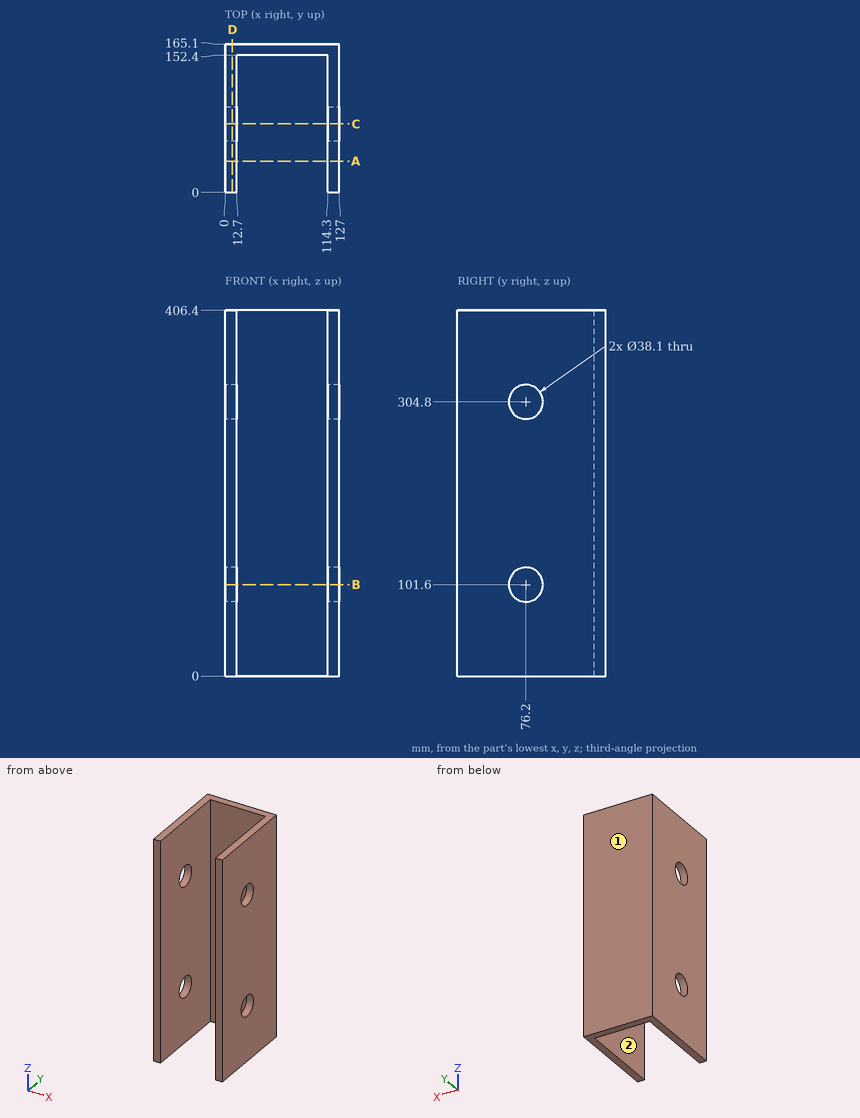
Study the drawing (mm; zero at the part's minimum x, y, z) and answer. A direction names the side the tool comes from. Give positions to 0.01 mm unless a question says otherwise; leave off trailing zeros. Loops run counter-clockwise (first coordinate to the right, second up) from the corner with the lowest first, then second, coordinate; pieces in that order, holes last. Notation, with made-up numbers: M 81.25,83 L 106.25,83 A9 cw 106.25,93 Z; hole C 73,66 d6. An arc over 180 degrees is marked long. Use CSV: the item, a comma, the result in double quotes.
1) Find section C-C on y = 76.2. Write down the section's boundary in (x, z), plus the area to 3 significant figures.
Answer:
outline,"M 0,0 L 12.7,0 L 12.7,82.55 L 0,82.55 Z; M 0,120.65 L 12.7,120.65 L 12.7,285.75 L 0,285.75 Z; M 0,323.85 L 12.7,323.85 L 12.7,406.4 L 0,406.4 Z; M 114.3,0 L 127,0 L 127,82.55 L 114.3,82.55 Z; M 114.3,120.65 L 127,120.65 L 127,285.75 L 114.3,285.75 Z; M 114.3,323.85 L 127,323.85 L 127,406.4 L 114.3,406.4 Z"
area,"8,390 mm^2"
2) Find section A-A on y = 35. Write down the section's boundary in (x, z).
Answer:
outline,"M 0,0 L 12.7,0 L 12.7,406.4 L 0,406.4 Z; M 114.3,0 L 127,0 L 127,406.4 L 114.3,406.4 Z"
3) Find section B-B on z = 101.6. Write down the section's boundary in (x, y), plus the area to 3 significant figures.
Answer:
outline,"M 0,0 L 12.7,0 L 12.7,57.15 L 0,57.15 Z; M 0,95.25 L 12.7,95.25 L 12.7,152.4 L 114.3,152.4 L 114.3,95.25 L 127,95.25 L 127,165.1 L 0,165.1 Z; M 114.3,0 L 127,0 L 127,57.15 L 114.3,57.15 Z"
area,"4,520 mm^2"
4) Which of the six approach directions +Z, -Z, +X, -X, +Y, -Y give full straight-line access (tool end or side, diameter ignored) to the marked faces 1 and 2?
Answer:
face 1,"+Z, -Z, +X, -X, +Y"
face 2,"+Z, -Z, -Y"
5) Consider L1, parallel to Z at x = 121.25, y = 76.2; L2, parallel to X at y = 147, z = 216; L3, parallel to Y at x = 37, z = 239.5. Determine where each line is inside the solid, lowest interval first.
Answer:
L1,"0 to 82.55, 120.65 to 285.75, 323.85 to 406.4"
L2,"0 to 12.7, 114.3 to 127"
L3,"152.4 to 165.1"
6) Find section D-D on x = 8. Write down the section's boundary in (y, z).
Answer:
outline,"M 0,0 L 165.1,0 L 165.1,406.4 L 0,406.4 Z; hole C 76.2,101.6 d38.1; hole C 76.2,304.8 d38.1"
